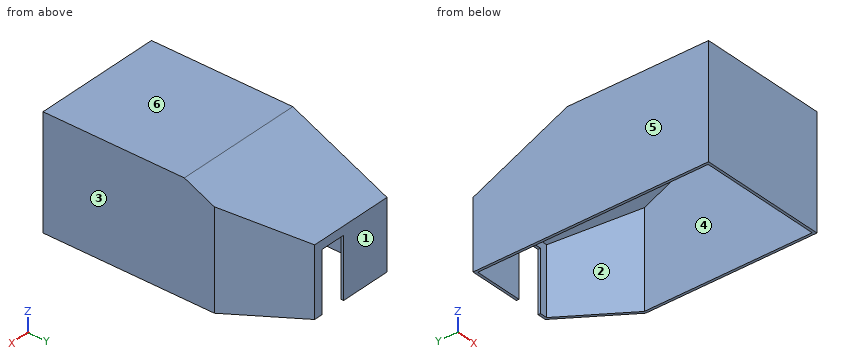
```python
from build123d import *

# Parameters (mm, degrees)
EXTRUDE_1_DEPTH     = 130
CHAMFER_1_SIZE      = 50
CHAMFER_1_SIZE2     = 110
SHELL_1_T           = -3
SKETCH_3_W          = 30
SKETCH_3_H          = 70
CUT_EXTRUDE_1_DEPTH = 3


with BuildPart() as part:
    # 草图2 → 凸台-拉伸1 (new body)
    with BuildSketch(Plane.XY):
        Polygon((-75, 280), (-75, 5), (75, 5), (75, 205), (25, 280), align=None)
    extrude(amount=EXTRUDE_1_DEPTH)

    # 倒角1
    chamfer_1_edges = [part.edges().sort_by_distance(p)[0] for p in [
        (-25, 280, 130),
    ]]
    chamfer_1_side = [part.faces().sort_by_distance(p)[0] for p in [
        (-25, 280, 65),
    ]]
    chamfer(chamfer_1_edges, length=CHAMFER_1_SIZE, length2=CHAMFER_1_SIZE2, reference=chamfer_1_side[0])

    # 抽壳1
    shell_1_openings = [part.faces().sort_by_distance(p)[0] for p in [
        (-2.777777778, 137.142857143, 0),
    ]]
    offset(amount=SHELL_1_T, openings=shell_1_openings, kind=Kind.INTERSECTION)

    # 草图3 → 切除-拉伸1 (cut)
    with BuildSketch(Plane(origin=(0, 280, 0), x_dir=(1, 0, 0), z_dir=(0, 1, 0))):
        with Locations((0, -35)):
            Rectangle(SKETCH_3_W, SKETCH_3_H)
    extrude(amount=-CUT_EXTRUDE_1_DEPTH, mode=Mode.SUBTRACT)


solid = part.part
```
Verification items for the finished model (mm, model axes). Face numbers are marked on the shaded views. A direction names the side the tool comes from. Round coordinates to 2 decimals unless told otherwise and drop trailing zeros. Write each loop counter-clockwise with the first axis right and the second up, starting at its lowest first coordinate (ties: lowest second). Pieces come first, ordered by that corner, then holes. Notation, with made-up numbers: (-14, 54.5) -> (35, 54.5) arc R22 cw to (35, 67.5) -> close; hole circle Ø10 at (7.5, 48.25). An arc over 180 degrees is marked (long way). Write each question's results on one line, items separated by ' | '.
Q1. Thickness scan on probe 1 along Y at (x, z) = (-62, 14.5); probe 2 along X at (y, z) = (139.5, 67); probe 3 along Z at (x, y) = (32, 24). Record the ranges inside material, lowest first.
Derived:
probe 1: y = 5 to 8, 277 to 280 | probe 2: x = -75 to -72, 72 to 75 | probe 3: z = 127 to 130
Q2. Sectioned sample at B-B, the plane z = 73.5. Record the boundary of the cut face in (x, y), and give its area (3 significant figures).
Derived:
outline: (-75, 5) -> (75, 5) -> (75, 205) -> (25, 280) -> (-75, 280) -> close; hole (-72, 8) -> (72, 8) -> (72, 204.09) -> (23.39, 277) -> (-72, 277) -> close | area: 2,410 mm²
Q3. Go/stop test with flat-tipped pins: pin 1 Ø0.9 at (y, z) = (278, 37.5) entering from +X; pin 2 Ø3.5 at (x, y) = (-5.5, 278.5) entering from -Z; pin 3 Ø5 at (x, y) = (-20, 138.5) entering from -Z. Record where each tip stops, or that it passes through.
Derived:
pin 1: stops at x = 26.63 | pin 2: stops at z = 70 | pin 3: stops at z = 127
Q4. Sectioned sample at A-A, the plane x = -50.5. Record the boundary of the cut face in (y, z), and give its area (3 significant figures).
Derived:
outline: (5, 0) -> (8, 0) -> (8, 127) -> (169.35, 127) -> (277, 78.07) -> (277, 0) -> (280, 0) -> (280, 80) -> (170, 130) -> (5, 130) -> close | area: 1,470 mm²
Q5. Sectioned sample at C-C, the plane y = 31.5. Record the boundary of the cut face in (x, z), and give its area (3 significant figures).
Derived:
outline: (-75, 0) -> (-72, 0) -> (-72, 127) -> (72, 127) -> (72, 0) -> (75, 0) -> (75, 130) -> (-75, 130) -> close | area: 1,210 mm²
Q6. Sectioned sample at D-D, the plane z = 9. Record the boundary of the cut face in (x, y), and give its area (3 significant figures).
Derived:
outline: (-75, 5) -> (75, 5) -> (75, 205) -> (25, 280) -> (15, 280) -> (15, 277) -> (23.39, 277) -> (72, 204.09) -> (72, 8) -> (-72, 8) -> (-72, 277) -> (-15, 277) -> (-15, 280) -> (-75, 280) -> close | area: 2,320 mm²
Q7. Draft check along X on the marked faces 3, 4, 5 and 6. Enter one of: released by +X, released by -X, zero draft, split by the parting line, or undercut.
Derived:
face 3: released by +X | face 4: undercut | face 5: released by -X | face 6: zero draft
Q8. Access from +Z, -Z, +X, -X, +Y, -Y to the whole of each face (thin tool, end or side, straight path). Record for the marked faces 1 and 2.
Derived:
face 1: +Z, -Z, +X, -X, +Y | face 2: -Z
